```python
from build123d import *

# Parameters (mm, degrees)
F0_W     = 76.2
F0_H     = 76.2
F1_DEPTH = 1.5875
F2_W     = 38.1
F2_H     = 38.1
F3_DEPTH = 25.4


# Not quite as in the source:
# - a length typed as a fraction of an inch, garbled in the dataset ("3 / 203.2 mm" for 3/8 in), is restored


with BuildPart() as f1:
    # F0 (on Right) → F1 (new body)
    with BuildSketch(Plane.YZ):
        Rectangle(F0_W, F0_H)
    extrude(amount=F1_DEPTH)

    # F2 (on face) → F3 (cut)
    with BuildSketch(Plane.YZ.offset(1.5875)):
        with Locations((19.05, 19.05)):
            Rectangle(F2_W, F2_H)
    extrude(amount=-F3_DEPTH, mode=Mode.SUBTRACT)


solid = f1.part
```
Here's how the part is built. I have some questions about the finished solid (model axes, mm). Round coordinates to 2 decimals unless told otherwise and drop trailing zeros. Write each loop counter-clockwise with the first axis right and the second up, starting at its lowest first coordinate (ties: lowest second). Pieces come first, ordered by that corner, then holes. Notation, with made-up numbers: M 36,50.5 L 51,50.5 A19 cw 51,65.5 Z; hole C 42.25,19 d5. An arc over 180 degrees is marked long. Answer as CSV lines item,"result". Start each with the question number.
1. Suppose I cut it at A-A on x = 0.6. Write out the boundary of the cut face in (y, z), then the cut area to 3 significant figures.
2. Suppose I cut it at B-B on y = 25.5. Write out the boundary of the cut face in (x, z), then the cut area to 3 significant figures.
3. I'm going to push a flat-ended pin straight in: pin 1 Ø0.8 at (x, y) = (1, 19.5) entering from +Z. Where does the tip first touch, or does it pass through?
4. I need wall thicknesses on probe 1 along Z at (x, y) = (0.5, 18.5). Which ranges of the line are inside material? Lowest first, please.
Check result:
1,outline,"M -38.1,-38.1 L 38.1,-38.1 L 38.1,0 L 0,0 L 0,38.1 L -38.1,38.1 Z"
1,area,"4,350 mm2"
2,outline,"M 0,-38.1 L 1.59,-38.1 L 1.59,0 L 0,0 Z"
2,area,"60.5 mm2"
3,pin 1,"stops at z = 0"
4,probe 1,"z = -38.1 to 0"
